Part print with two shaded views. Sizes in mm from the minimum x, y, z corner. A direction names the side the tool comes from. Round coordinates to 2 decimals unless told otherwise and drop trailing zeros. Order: outer loops, then holes, each group sorted by start corner. A loop starts at its lowest first (then second) coordinate and runs counter-clockwise, first axis right, second up. Notation, with made-up numbers: (-31, 40) -> (10, 40) arc R26 cw to (10, 69) -> close; hole circle Ø10 at (55.5, 69.5). An arc over 180 degrees is marked (long way). Use a Markdown table: item, result. Add a question column.
Item 1: Pin check, flat tip, straight feed: pin 1 (1.8 mm diameter, centred on x = 35.5, z = 3.5, fed in from -Y). Stop position of the tip, or through.
Item 2: Slice it at B-B, the plane z = 4.3. State how many separate pieces and enclosed holes the cut face has, plus the area to 3 significant figures.
Item 3: Slice it at D-D, the plane x = 13.5. Give the cut face in (y, z).
Item 4: Slice it at C-C, the plane y = 12.7. Give the cut face in (x, z) (1 decimal).
Item 5: Two-plate mould, pull along X, no slides. Class the marked faces 4, 5, 6 and 7: released by +X, released by -X, zero draft, split by the parting line, or undercut.
Item 6: Slice it at A-A, the plane y = 20.5. Give the cut face in (x, z) (1 decimal).
Item 7: 3-axis set-ups, long thin cutter, end or side, ignore diameter. For the marked faces 1, 2 and 3: which of +Z, -Z, +X, -X, +Y, -Y reach the whole face in a straight line?
Item 8: Probe L1, parallel to X at y = 2, z = 0.55 (1 decimal); L2, parallel to X at y = 14, z = 0.95; L3, parallel to X at y = 11.75, z = 2.55. List the from-to ranges inside material, lowest first.
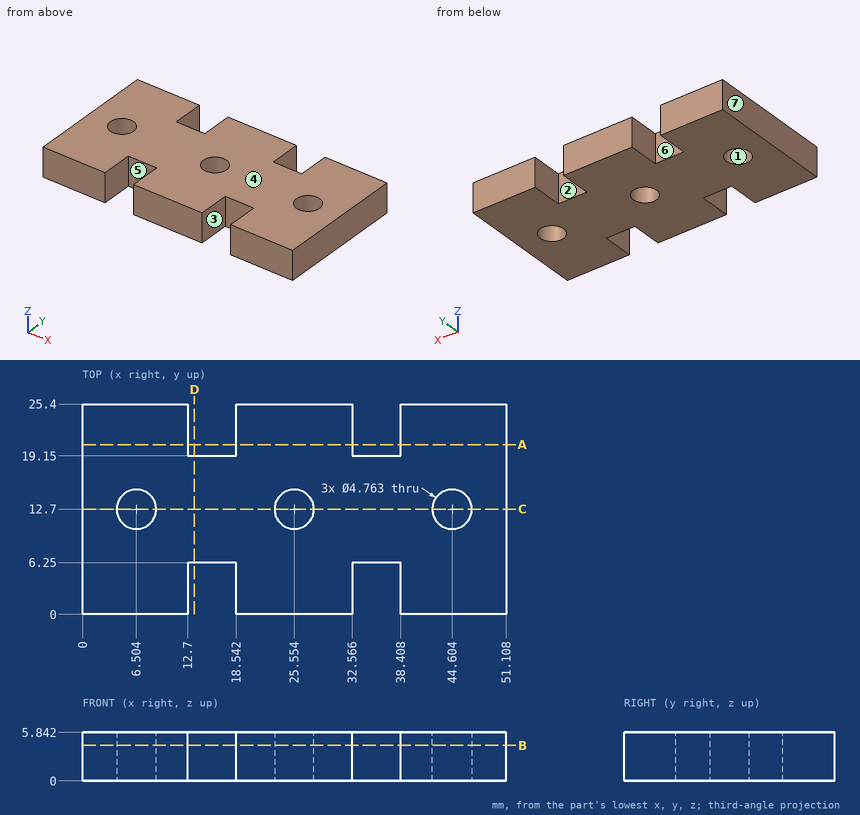
Check sheet entries:
| question | item | result |
|---|---|---|
| 1 | pin 1 | y = 6.25 |
| 2 | separate pieces | 1 |
| 2 | enclosed holes | 3 |
| 2 | area | 1,100 mm2 |
| 3 | outline | (6.25, 0) -> (19.15, 0) -> (19.15, 5.84) -> (6.25, 5.84) -> close |
| 4 | outline | (0, 0) -> (4.1, 0) -> (4.1, 5.8) -> (0, 5.8) -> close; (8.9, 0) -> (23.2, 0) -> (23.2, 5.8) -> (8.9, 5.8) -> close; (27.9, 0) -> (42.2, 0) -> (42.2, 5.8) -> (27.9, 5.8) -> close; (47, 0) -> (51.1, 0) -> (51.1, 5.8) -> (47, 5.8) -> close |
| 5 | face 4 | zero draft |
| 5 | face 5 | undercut |
| 5 | face 6 | undercut |
| 5 | face 7 | released by -X |
| 6 | outline | (0, 0) -> (12.7, 0) -> (12.7, 5.8) -> (0, 5.8) -> close; (18.5, 0) -> (32.6, 0) -> (32.6, 5.8) -> (18.5, 5.8) -> close; (38.4, 0) -> (51.1, 0) -> (51.1, 5.8) -> (38.4, 5.8) -> close |
| 7 | face 1 | +Z, -Z |
| 7 | face 2 | +Z, -Z, +Y |
| 7 | face 3 | +Z, -Z, -Y |
| 8 | L1 | 0 to 12.7, 18.5 to 32.6, 38.4 to 51.1 |
| 8 | L2 | 0 to 4.51, 8.5 to 23.56, 27.55 to 42.61, 46.6 to 51.11 |
| 8 | L3 | 0 to 4.32, 8.69 to 23.37, 27.74 to 42.42, 46.79 to 51.11 |
